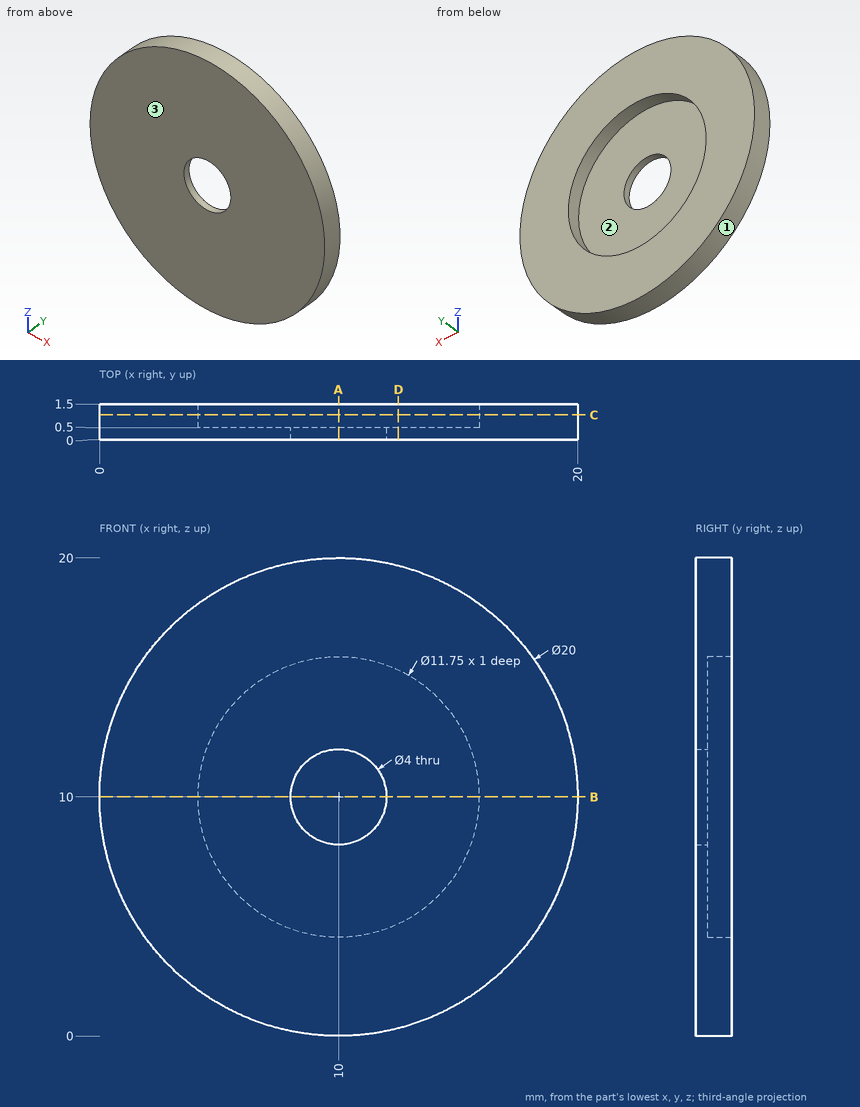
For this review, use the dimensioned drawing (mm, ordinates from the lowest corner) and the shaded views. Give positions to 0.01 mm unless a question says otherwise; leave off trailing zeros. Order: outer loops, then holes, each group sorted by start corner. A loop starts at its lowest first (then second) coordinate and runs counter-clockwise, first axis right, second up. Notation, with made-up numbers: M -35.75,43 L 23.25,43 A24 cw 23.25,70 Z; hole C -9,-9 d1. An arc over 180 degrees is marked long. Use one line per item in the form item = value. Start each with the question number.
Item 1: Insertion check: pin 1 Ø10.5 at (x, z) = (10, 10) entering from +Y; pin 2 Ø5 at (x, z) = (3.5, 4.5) entering from -Y. Each pin has a flat end and moves straight along its axis. Give the tip position at first contact, or say it passes through.
Item 2: We need section C-C on y = 1.05. Give the boundary of the cut face in (x, z) (3 decimals).
Item 3: The part is to be moulded in two halves that separate along Z. For the marked faces 1, 2 and 3, say which applies: pulls with the +Z half, pulls with the -Z half, needs draft (parallel to the pull), parting line crosses it, or undercut.
Item 4: We need section D-D on x = 12.5. Give the boundary of the cut face in (y, z).
Item 5: We need section B-B on z = 10. Give the boundary of the cut face in (x, y) (3 decimals).
Item 6: We need section A-A on x = 10. Give the boundary of the cut face in (y, z) (3 decimals).
Item 7: To check wall thickness, follow line 1 along Z through (x, y) = (10, 1.2) (3 decimals); line 2 along Z through (x, y) = (10, 0.15); line 3 along Y through (x, z) = (11, 14). State the ranges of each line that lie inside material, in increasing order. Write a range as from..to.
Completed:
q1.pin_1 = 0.5
q1.pin_2 = 0
q2.outline = C 10,10 d20; hole C 10,10 d11.75
q3.face_1 = parting line crosses it
q3.face_2 = undercut
q3.face_3 = needs draft
q4.outline = M 0,0.32 L 1.5,0.32 L 1.5,4.68 L 0.5,4.68 L 0.5,15.32 L 1.5,15.32 L 1.5,19.68 L 0,19.68 Z
q5.outline = M 0,0 L 8,0 L 8,0.5 L 4.125,0.5 L 4.125,1.5 L 0,1.5 Z; M 12,0 L 20,0 L 20,1.5 L 15.875,1.5 L 15.875,0.5 L 12,0.5 Z
q6.outline = M 0,0 L 1.5,0 L 1.5,4.125 L 0.5,4.125 L 0.5,8 L 0,8 Z; M 0,12 L 0.5,12 L 0.5,15.875 L 1.5,15.875 L 1.5,20 L 0,20 Z
q7.line_1 = 0..4.125, 15.875..20
q7.line_2 = 0..8, 12..20
q7.line_3 = 0..0.5
